```python
from build123d import *

# Parameters (mm, degrees)
SKETCH1_W             = 40
SKETCH1_H             = 50
BOSS_EXTRUDE1_DEPTH   = 10
SKETCH2_W             = 40
SKETCH2_H             = 5
BOSS_EXTRUDE2_DEPTH   = 40
F_2_0MM_DOWEL_HOLE1_D = 2
FILLET1_R             = 10


with BuildPart() as part:
    # Sketch1 → Boss-Extrude1 (new body)
    with BuildSketch(Plane(origin=(0, 0, 0), x_dir=(1, 0, 0), z_dir=(0, 1, 0))):
        Rectangle(SKETCH1_W, SKETCH1_H)
    extrude(amount=BOSS_EXTRUDE1_DEPTH)

    # Sketch2 → Boss-Extrude2 (add)
    with BuildSketch(Plane(origin=(0, 10, 0), x_dir=(1, 0, 0), z_dir=(0, 1, 0))):
        with Locations((0, -22.5)):
            Rectangle(SKETCH2_W, SKETCH2_H)
    extrude(amount=BOSS_EXTRUDE2_DEPTH)

    # Ø2.0mm Dowel Hole1 (through all)
    with Locations(Plane.XY.offset(25)):
        with Locations((-10.5, 38), (10.5, 38), (-10.5, 25.5), (10.5, 25.5)):
            Hole(F_2_0MM_DOWEL_HOLE1_D / 2)

    # Fillet1
    fillet1_edges = [part.edges().sort_by_distance(p)[0] for p in [
        (0, 10, 20),
        (-20, 50, 22.5),
        (20, 50, 22.5),
    ]]
    fillet(fillet1_edges, radius=FILLET1_R)


solid = part.part
```
Build history of the part. All positions in model axes, mm. A direction names the side the tool comes from. Round coordinates to 2 decimals unless told otherwise and drop trailing zeros. Order: outer loops, then holes, each group sorted by start corner. A loop starts at its lowest first (then second) coordinate and runs counter-clockwise, first axis right, second up. Notation, with made-up numbers: (21.5, 68.5) -> (36.5, 68.5) arc R24 cw to (36.5, 101.5) -> close; hole circle Ø11 at (-12.5, 36.25). An arc over 180 degrees is marked (long way). Answer in a Markdown table with one row per item.
1) Wall check: L1, parallel to Y at x = 10.5, z = 21.4; L2, parallel to Z at x = 16.5, y = 35; L3, parallel to Y at x = -2, z = 0. Give the ranges that are in metal, low to high.
Values:
| item | result |
|---|---|
| L1 | 0 to 24.5, 26.5 to 37, 39 to 49.99 |
| L2 | 20 to 25 |
| L3 | 0 to 10 |
2) Band-saw the part on D-D on y = 16. Give the cut face in (x, z), and give its area (3 significant figures).
Values:
| item | result |
|---|---|
| outline | (-20, 19.17) -> (20, 19.17) -> (20, 25) -> (-20, 25) -> close |
| area | 233 mm2 |
3) Band-saw the part on A-A on y = 25.5. Give the cut face in (x, z), and give its area (3 significant figures).
Values:
| item | result |
|---|---|
| outline | (-20, 20) -> (-11.5, 20) -> (-11.5, 25) -> (-20, 25) -> close; (-9.5, 20) -> (9.5, 20) -> (9.5, 25) -> (-9.5, 25) -> close; (11.5, 20) -> (20, 20) -> (20, 25) -> (11.5, 25) -> close |
| area | 180 mm2 |
4) Which spindle directions (+Z, -Z, +X, -X, +Y, -Y) get a long thin tool onto all of the face, cutting with end or side? Do faces 4 (the cylindrical face through (10.717, 24.524, 22.465)), 5 (the flat face through (0, 10, -8)). Say none if no direction does.
Values:
| item | result |
|---|---|
| face 4 | +Z, -Z |
| face 5 | -Z, +X, -X, +Y |
5) Band-saw the part on B-B on x = 4.5. Give the cut face in (y, z).
Values:
| item | result |
|---|---|
| outline | (0, -25) -> (10, -25) -> (10, 10) arc R10 cw to (20, 20) -> (50, 20) -> (50, 25) -> (0, 25) -> close |
6) Mould opens along X. For faces 1 (the flat face through (0, 50, 22)), 2 (the cylindrical face through (16.99, 47.15, 22.46)), 3 (the cylindrical face through (10.63, 38.99, 22.47)) say: released by +X, released by -X, zero draft, split by the parting line, or undercut.
Values:
| item | result |
|---|---|
| face 1 | zero draft |
| face 2 | released by +X |
| face 3 | undercut |
7) Pin check, flat tips, straight feed: P1, Ø1.5, axis at x = -15, y = 39.5, coming from the -Z side; P2, Ø1, axis at x = -14, y = 17.5, coming from the -Z side; P3, Ø3, axis at x = -15.5, y = 19.5, coming from the -Z side; P4, Ø1.6, axis at x = -10.5, y = 38, coming from the -Z side. Stop position of each tip, or through.
Values:
| item | result |
|---|---|
| P1 | z = 20 |
| P2 | z = 19.54 |
| P3 | z = 19.8 |
| P4 | through |
8) Band-saw the part on C-C on z = -5. Give the cut face in (x, y), and give its area (3 significant figures).
Values:
| item | result |
|---|---|
| outline | (-20, 0) -> (20, 0) -> (20, 10) -> (-20, 10) -> close |
| area | 400 mm2 |
